Autodesk Inventor part; units mm, degrees
ref_plane "YZ Plane" through (0, 0, 0) normal (1, 0, 0) x (0, 1, 0)
ref_plane "XZ Plane" through (0, 0, 0) normal (0, 1, 0) x (-1, 0, 0)
ref_plane "XY Plane" through (0, 0, 0) normal (0, 0, 1) x (1, 0, 0)
sketch "Sketch1" plane through (0, 0, 0) normal (0, 0, 1) x (1, 0, 0)
  line L0 (0, 23) -> (-1.087, 23)
  line L1 (-1.587, 22.5) -> (-1.587, 0)
  line L2 (0, 23) -> (0, -11)
  line L3 (0, -11) -> (0, -10.95)
  line L4 (0, -11) -> (-0.05, -11)
  line L5 (-0.05, -11) -> (-1.587, 0)
  arc A0 (-1.087, 23) -> (-1.587, 22.5) centre (-1.087, 22.5) ccw
  point P0 (-1.587, 23)
  dimension "d1" = 1.587
  dimension "d8" = 0.05
  dimension "d13" = 0.5
revolve "Revolution1" add sketch "Sketch1" angle 360 about axis through (0, 23, 0) along (0, -1, 0)
sketch "Sketch2" plane through (0, -11, 0) normal (0, -1, 0) x (1, 0, 0)
  line L0 (0.05, 1.7032) -> (0.05, -1.887)
  line L1 (0.05, -1.887) -> (1.6041, -1.887)
  line L2 (1.6041, -1.887) -> (1.6041, 1.7032)
  line L3 (1.6041, 1.7032) -> (0.05, 1.7032)
  point P0 (0, 0)
  dimension "d10" = 0.05
extrude "Extrusion1" cut sketch "Sketch2" against normal blind 11
fillet "Fillet1" radius 0.65 1 edges at (0.05, 0, 0)
properties part number "Herramienta Punta de Lanza"
Here's how the part is built. I have some questions about the finished solid (model axes, mm). A direction names the side the tool comes from. Coordinates: 2 decimals unless noted, no trailing zeros. Write each loop counter-clockwise with the first axis right and the second up, starting at its lowest first coordinate (ties: lowest second). Pieces come first, ordered by that corner, then holes. Notation, with made-up numbers: (56.5, -0.5) - (105.5, -0.5) arc R9 ccw to (105.5, 13.5) - close; hole circle Ø3 at (78.25, 82). An arc over 180 degrees is marked (long way). One line per item, written item: value.
1) Suppose I cut it at A-A on y = 18. Write out the boundary of the cut face in (x, z), and give its area (3 significant figures).
Model answer:
outline: circle Ø3.17 at (0, 0)
area: 7.91 mm²
2) I need wall thicknesses on line 1 along Z through (x, y) = (-0.7, 9.5); line 2 along X through (y, z) = (-5, -0.6); line 3 along Y through (x, z) = (0.95, -0.45). Which ranges of each line are inside material? Lowest first, please.
Model answer:
line 1: z = -1.42 to 1.42
line 2: x = -0.66 to 0.05
line 3: y = 0 to 23
3) On a 3-axis mill with a long thin cutter (end or side, diameter ignored), from which of +Z, -Z, +X, -X, +Y, -Y can I reach the whole of each face in a straight line? I mean faces 1 (the flat face through (0, 23, 0)), 2 (the flat face through (1, 0, 0)). Say none if no direction works.
Model answer:
face 1: +Z, -Z, +X, -X, +Y
face 2: +Z, -Z, +X, -Y
4) I'm going to push a flat-ended pin straight in: P1, Ø0.9, axis at y = -6.5, z = 0.5, coming from the +X side. Where does the tip first touch, or does it pass through?
Model answer:
P1: stops at x = 0.05
